Autodesk Inventor part; units mm, degrees
ref_plane "YZ Plane" through (0, 0, 0) normal (1, 0, 0) x (0, 1, 0)
ref_plane "XZ Plane" through (0, 0, 0) normal (0, 1, 0) x (-1, 0, 0)
ref_plane "XY Plane" through (0, 0, 0) normal (0, 0, 1) x (1, 0, 0)
sketch "Skizze1" plane through (0, 0, 0) normal (0, 0, 1) x (1, 0, 0)
  line L0 (0, 2.8868) -> (2.5, 1.4434)
  line L1 (2.5, 1.4434) -> (2.5, -1.4434)
  line L2 (2.5, -1.4434) -> (0, -2.8868)
  line L3 (0, -2.8868) -> (-2.5, -1.4434)
  line L4 (-2.5, -1.4434) -> (-2.5, 1.4434)
  line L5 (-2.5, 1.4434) -> (0, 2.8868)
  circle A0 centre (0, 0) radius 1.5
  dimension "d0" = 5
  dimension "d1" = 3
extrude "Extrusion1" add sketch "Skizze1" along normal blind 5
chamfer "Fase1" distance 0.3 angle 45 13 edges at (1.25, -2.1651, 5) (-1.25, -2.1651, 5) (2.5, 0, 5) (1.25, 2.1651, 5) (-1.25, 2.1651, 5) (1.25, -2.1651, 0) (2.5, 0, 0) (-1.25, -2.1651, 0) (1.25, 2.1651, 0) (-1.25, 2.1651, 0) (-2.5, 0, 0) (-1.5, 0, 5) (-1.5, 0, 0)
thread "Gewinde1"
sketch "Skizze2" plane through (0, 0, 5) normal (0, 0, 1) x (1, 0, 0)
  line L0 (0, -2.5403) -> (-2.5, -1.097)
  line L1 (2.2, -1.2702) -> (0, -2.5403)
  line L2 (2.2, 1.2702) -> (2.2, -1.2702)
  line L3 (0, 2.5403) -> (2.2, 1.2702)
  line L4 (-2.5, 1.097) -> (0, 2.5403)
  line L5 (-2.5, 1.097) -> (-2.5, -1.097)
  circle A0 centre (0, 0) radius 1.8
extrude "Extrusion2" add sketch "Skizze2" against normal blind 1 contours A0
sketch "Skizze3" plane through (0, 0, 5) normal (0, 0, 1) x (1, 0, 0)
  circle A0 centre (0, 0) radius 1.5
  dimension "d11" = 3
extrude "Extrusion3" add sketch "Skizze3" along normal blind 5
thread "Gewinde2"
chamfer "Fase2" distance 0.3 angle 45 1 edges at (-1.5, 0, 10)
properties part number "Distanzhuelse_M3x5mm_" material "Nickel-Kupfer-Legierung 400"
Check sheet for the modelled part. Datum: model origin and axes. Units: mm. A direction names the side the tool comes from. Coordinates: 2 decimals unless noted, no trailing zeros. Order: outer loops, then holes, each group sorted by start corner. A loop starts at its lowest first (then second) coordinate and runs counter-clockwise, first axis right, second up. Notation, with made-up numbers: M 37,25.5 L 79,25.5 A24 ccw 79,44.5 Z; hole C -34.5,37.5 d5. An arc over 180 degrees is marked long. Write each question's results on one line, items separated by ' | '. Start each with the question number.
1. Go/stop test with flat-tipped pins: P1, Ø1.4, axis at x = 0.5, y = 1.5, coming from the +Z side; P2, Ø2.5, axis at x = 0, y = 0.5, coming from the -Z side; P3, Ø2, axis at y = 0, z = 7, coming from the +X side; P4, Ø2, axis at y = -1.5, z = 8, coming from the -X side. Record where each tip stops, or that it passes through.
2. Cross-section at C-C on z = 4.5. Record the cut outline in (x, y), and give its area (3 significant figures).
3. Access from +Z, -Z, +X, -X, +Y, -Y to the whole of each face (thin tool, end or side, straight path). Record for faces 1 (the face through (0, 0, 10)), 2 (the face through (-1.2, 1.2, 5)).
4. Mould release check, pull along Y, two halves, no side actions. Record for faces 3 (the face through (-1.5, -0.07, 2.12)), 4 (the face through (-1.233, -2.175, 2.469)), 5 (the face through (-1.5, -0.07, 7.32)), 6 (the face through (1.191, 2.023, 0.148)): +Y half, -Y half, draft (parallel to the pull), parting line (faces both ways), or undercut.
5. Cross-section at A-A on y = 0. Record the cut outline in (x, z), and give its area (3 significant figures).
6. Material ranges on probe 1 along X at (y, z) = (0.1, 2.75); probe 2 along Z at (x, y) = (-1.25, -1.35); probe 3 along Z at (x, y) = (0.2, 0.2), recorded low to high.
7. Cross-section at B-B on z = 1.75. Record the cut outline in (x, y), and give its area (3 significant figures).
Checks:
1) P1: stops at z = 10 | P2: stops at z = 0.05 | P3: stops at x = 1.5 | P4: stops at x = -1.41
2) outline: M -2.5,-1.44 L 0,-2.89 L 2.5,-1.44 L 2.5,1.44 L 0,2.89 L -2.5,1.44 Z | area: 21.7 mm²
3) face 1: +Z, +X, -X, +Y, -Y | face 2: +Z
4) face 3: undercut | face 4: -Y half | face 5: parting line | face 6: +Y half
5) outline: M -2.5,0.3 L -2.2,0 L -1.8,0 L -1.5,0.3 L -1.5,4 L 1.5,4 L 1.5,0.3 L 1.8,0 L 2.2,0 L 2.5,0.3 L 2.5,4.7 L 2.2,5 L 1.5,5 L 1.5,9.7 L 1.2,10 L -1.2,10 L -1.5,9.7 L -1.5,5 L -2.5,5 Z | area: 27.7 mm²
6) probe 1: x = -2.5 to -1.5, 1.5 to 2.5 | probe 2: z = 0 to 5 | probe 3: z = 4 to 10
7) outline: M -2.5,-1.44 L 0,-2.89 L 2.5,-1.44 L 2.5,1.44 L 0,2.89 L -2.5,1.44 Z; hole C 0,0 d3 | area: 14.6 mm²
